Autodesk Inventor part; units mm, degrees
ref_plane "YZ Plane" through (0, 0, 0) normal (1, 0, 0) x (0, 1, 0)
ref_plane "XZ Plane" through (0, 0, 0) normal (0, 1, 0) x (-1, 0, 0)
ref_plane "XY Plane" through (0, 0, 0) normal (0, 0, 1) x (1, 0, 0)
sketch "Sketch1" plane through (0, 0, 0) normal (0, 0, 1) x (1, 0, 0)
  line L0 (0, 0) -> (180, 0)
  line L1 (180, 0) -> (180, 170)
  line L2 (180, 170) -> (0, 170)
  line L3 (0, 170) -> (0, 0)
  line L4 (0, 40) -> (-5, 40)
  line L5 (-5, 40) -> (-5, 90)
  line L6 (-5, 90) -> (0, 90)
  line L7 (0, 90) -> (0, 40)
  line L8 (90, 0) -> (90, 170) construction
  line L9 (180, 40) -> (185, 40)
  line L10 (185, 40) -> (185, 90)
  line L11 (185, 90) -> (180, 90)
  line L12 (180, 90) -> (180, 40)
  line L13 (30, 105) -> (150, 105)
  line L14 (150, 105) -> (150, 110)
  line L15 (150, 110) -> (30, 110)
  line L16 (30, 110) -> (30, 105)
  line L17 (0, 65) -> (180, 65) construction
  line L18 (40, 170) -> (140, 170)
  line L19 (140, 170) -> (140, 175)
  line L20 (140, 175) -> (40, 175)
  line L21 (40, 175) -> (40, 170)
  point P0 (180, 40)
  point P1 (180, 90)
  point P2 (0, 90)
  point P3 (40, 0)
  point P4 (30, 107.5)
  dimension "d0" = 180
  dimension "d1" = 170
  dimension "d2" = 5
  dimension "d3" = 50
  dimension "d6" = 120
  dimension "d7" = 5
  dimension "d13" = 60
  dimension "d14" = 60
  dimension "d30" = 100
  dimension "d31" = 5
  dimension "d32" = 40
extrude "Extrusion1" add sketch "Sketch1" along normal blind 5
sketch "Sketch2" plane through (0, 0, 5) normal (0, 0, 1) x (1, 0, 0)
  line L0 (180, 170) -> (0, 170)
  line L1 (0, 0) -> (180, 0)
  line L2 (0, 170) -> (0, 90)
  line L3 (0, 40) -> (0, 0)
  point P0 (85, 15)
  point P1 (95, 15)
  dimension "d24" = 15
  dimension "d25" = 15
  dimension "d26" = 10
  dimension "d29" = 85
hole "Hole1" at (85, 15, 5) at (95, 15, 5) direction (0, 0, -1) diameter 4 end through all
sketch "Sketch3" plane through (0, 0, 5) normal (0, 0, 1) x (1, 0, 0)
  line L0 (140, 175) -> (40, 175)
  line L1 (40, 175) -> (40, 170)
  point P0 (0, 0)
  point P1 (85, 155)
  point P2 (95, 155)
  dimension "d40" = 20
  dimension "d41" = 20
  dimension "d42" = 10
  dimension "d43" = 45
hole "Hole2" at (85, 155, 5) at (95, 155, 5) direction (0, 0, -1) diameter 4 end through all
properties part number "back"
Work out the finished part from the listing and answer in its coordinate system (mm). A direction names the side the tool comes from. Give positions to 0.01 mm unless a question says otherwise; leave off trailing zeros. Loops run counter-clockwise (first coordinate to the right, second up) from the corner with the lowest first, then second, coordinate; pieces in that order, holes last. Notation, with made-up numbers: M -13,74.25 L 2,74.25 A19 cw 2,99.25 Z; hole C -29.5,-9.5 d7. An arc over 180 degrees is marked long. One line per item, written item: value. Start each with the question number.
1. Each of these flat-tipped pins is pushed along its axis until it touches: P1, Ø1.5, axis at y = 115, z = 1.5, coming from the -X side; P2, Ø3, axis at y = 19.5, z = 3.5, coming from the +X side; P3, Ø2.5, axis at x = 85, y = 155, coming from the +Z side; P4, Ø2.5, axis at x = -3, z = 3, coming from the +Y side. Where does it stop, or does it pass through?
2. Find the intervals of material crossed by probe 1 along X at (y, z) = (15, 1.45); probe 2 along Y at (x, z) = (95, 3.4); probe 3 along Y at (x, z) = (58.5, 0.55), in increasing order.
3. Find section B-B (z = 1.2). Give the vertices of the cut face in (x, y), and give its area (3 significant figures).
4. Find section A-A (x = 107). Give the vertices of the cut face in (y, z).
5. Which of the six approach directions +Z, -Z, +X, -X, +Y, -Y give full straight-line access (tool end or side, diameter ignored) to faces 4 (the face through (0, 20, 2)), 5 (the face through (180, 20, 2)), 6 (the face through (140, 172, 2))?
6. Find section C-C (y = 35). Give the vertices of the cut face in (x, z).
7. Determine the mould class of faces 1 (the face through (160, 170, 2)), 2 (the face through (89, 105, 2)), 3 (the face through (89, 0, 2)) for opening direction Y: released by +Y, released by -Y, zero draft, split by the parting line, or undercut.
Reported:
1. P1: stops at x = 0
1. P2: stops at x = 180
1. P3: passes through
1. P4: stops at y = 90
2. probe 1: x = 0 to 83, 87 to 93, 97 to 180
2. probe 2: y = 0 to 13, 17 to 105, 110 to 153, 157 to 175
2. probe 3: y = 0 to 105, 110 to 175
3. outline: M -5,40 L 0,40 L 0,0 L 180,0 L 180,40 L 185,40 L 185,90 L 180,90 L 180,170 L 140,170 L 140,175 L 40,175 L 40,170 L 0,170 L 0,90 L -5,90 Z; hole M 30,105 L 150,105 L 150,110 L 30,110 Z; hole C 85,15 d4; hole C 85,155 d4; hole C 95,15 d4; hole C 95,155 d4
3. area: 30,900 mm²
4. outline: M 0,0 L 105,0 L 105,5 L 0,5 Z; M 110,0 L 175,0 L 175,5 L 110,5 Z
5. face 4: +Z, -Z, -X, -Y
5. face 5: +Z, -Z, +X, -Y
5. face 6: +Z, -Z, +X, +Y
6. outline: M 0,0 L 180,0 L 180,5 L 0,5 Z
7. face 1: released by +Y
7. face 2: undercut
7. face 3: released by -Y
